Here's how the part is built. I have some questions about the finished solid (model axes, mm). A direction names the side the tool comes from. Coordinates: 2 decimals unless noted, no trailing zeros. Write each loop counter-clockwise with the first axis right and the second up, starting at its lowest first coordinate (ties: lowest second). Pieces come first, ordered by that corner, then holes. Notation, with made-up numbers: M 13.5,27.25 L 69.5,27.25 A31 ccw 69.5,58.25 Z; hole C 14.25,1.5 d4. An arc over 180 degrees is marked long. Use one line per item in the form item = value. Start each with the question number.
1. I want a section at A-A, the plane y = 3. List the corners of the cut face in (x, z) for me, plus the area to 3 significant figures.
2. Thinking about a two-plate mould opening in Y: for faces 1 (the face through (35.6, 25.926, 0)), 2 (the face through (40, 8, 0)), 3 (the face through (32, 0, 0)), which applies, released by +Y, released by -Y, zero draft, split by the parting line, or undercut?
3. I want a section at D-D, the plane x = 27. List the corners of the cut face in (y, z) for me.
4. On a 3-axis mill with a long thin cutter (end or side, diameter ignored), from which of +Z, -Z, +X, -X, +Y, -Y can I reach the whole of each face in a straight line? I mean faces 4 (the face through (38, 15.926, 0)), 5 (the face through (4.926, 25, 0)), 6 (the face through (20, 20, -1.5)). Say none if no direction works.
5. I'm going to push a flat-ended pin straight in: pin 1 Ø1.5 at (y, z) = (22.5, 0) entering from +X. Where does the tip first touch, or does it pass through?
6. Please list where these lines run through material, in increasing order: line 1 along Y through (x, z) = (4.5, 0.7); line 2 along Y through (x, z) = (15, -1.25); line 3 along X through (y, z) = (33, -1.25). Write a range as [from, to].
7. I want a section at B-B, the plane x = 32. List the corners of the cut face in (y, z) for me, plus the area to 3 significant figures.
8. I want a section at C-C, the plane y = 27. List the corners of the cut face in (x, z) for me, plus the area to 3 significant figures.
Autodesk Inventor part; units mm, degrees
ref_plane "YZ Plane" through (0, 0, 0) normal (1, 0, 0) x (0, 1, 0)
ref_plane "XZ Plane" through (0, 0, 0) normal (0, 1, 0) x (-1, 0, 0)
ref_plane "XY Plane" through (0, 0, 0) normal (0, 0, 1) x (1, 0, 0)
sketch "스케치1" plane through (0, 0, 0) normal (0, 0, 1) x (1, 0, 0)
  line L0 (40, 40) -> (25, 40)
  line L1 (15, 40) -> (0, 40)
  line L2 (16, 40) -> (16, 35)
  line L3 (16, 35) -> (14, 35)
  line L4 (14, 35) -> (14, 36)
  line L5 (14, 36) -> (11, 36)
  line L6 (11, 36) -> (11, 31)
  line L7 (11, 31) -> (14, 28)
  line L8 (11, 31) -> (20.81, 31) construction
  line L9 (14, 28) -> (20, 28)
  line L10 (24, 40) -> (24, 35)
  line L11 (24, 35) -> (26, 35)
  line L12 (26, 35) -> (26, 36)
  line L13 (26, 36) -> (29, 36)
  line L14 (29, 36) -> (29, 31)
  line L15 (29, 31) -> (26, 28)
  line L16 (29, 31) -> (19.19, 31) construction
  line L17 (26, 28) -> (20, 28)
  line L18 (-0.0744, 15.9256) -> (4.9256, 15.9256)
  line L19 (-0.0744, 23.9256) -> (4.9256, 23.9256)
  line L20 (4.9256, 23.9256) -> (4.9256, 25.9256)
  line L21 (11.9256, 25.9256) -> (11.9256, 19.9256)
  line L22 (8.9256, 28.9256) -> (8.9256, 19.1155) construction
  line L23 (8.9256, 28.9256) -> (11.9256, 25.9256)
  line L24 (3.9256, 28.9256) -> (8.9256, 28.9256)
  line L25 (3.9256, 25.9256) -> (3.9256, 28.9256)
  line L26 (4.9256, 25.9256) -> (3.9256, 25.9256)
  line L27 (4.9256, 15.9256) -> (4.9256, 13.9256)
  line L28 (11.9256, 13.9256) -> (11.9256, 19.9256)
  line L29 (4.9256, 13.9256) -> (3.9256, 13.9256)
  line L30 (8.9256, 10.9256) -> (11.9256, 13.9256)
  line L31 (8.9256, 10.9256) -> (8.9256, 20.7356) construction
  line L32 (3.9256, 13.9256) -> (3.9256, 10.9256)
  line L33 (3.9256, 10.9256) -> (8.9256, 10.9256)
  line L34 (24, -0.1488) -> (24, 4.8512)
  line L35 (16, -0.1488) -> (16, 4.8512)
  line L36 (16, 4.8512) -> (14, 4.8512)
  line L37 (14, 11.8512) -> (20, 11.8512)
  line L38 (11, 8.8512) -> (20.81, 8.8512) construction
  line L39 (11, 8.8512) -> (14, 11.8512)
  line L40 (11, 3.8512) -> (11, 8.8512)
  line L41 (14, 3.8512) -> (11, 3.8512)
  line L42 (14, 4.8512) -> (14, 3.8512)
  line L43 (24, 4.8512) -> (26, 4.8512)
  line L44 (26, 11.8512) -> (20, 11.8512)
  line L45 (26, 4.8512) -> (26, 3.8512)
  line L46 (29, 8.8512) -> (26, 11.8512)
  line L47 (29, 8.8512) -> (19.19, 8.8512) construction
  line L48 (26, 3.8512) -> (29, 3.8512)
  line L49 (29, 3.8512) -> (29, 8.8512)
  line L50 (40.0744, 23.9256) -> (35.0744, 23.9256)
  line L51 (40.0744, 15.9256) -> (35.0744, 15.9256)
  line L52 (35.0744, 15.9256) -> (35.0744, 13.9256)
  line L53 (28.0744, 13.9256) -> (28.0744, 19.9256)
  line L54 (31.0744, 10.9256) -> (31.0744, 20.7356) construction
  line L55 (31.0744, 10.9256) -> (28.0744, 13.9256)
  line L56 (36.0744, 10.9256) -> (31.0744, 10.9256)
  line L57 (36.0744, 13.9256) -> (36.0744, 10.9256)
  line L58 (35.0744, 13.9256) -> (36.0744, 13.9256)
  line L59 (35.0744, 23.9256) -> (35.0744, 25.9256)
  line L60 (28.0744, 25.9256) -> (28.0744, 19.9256)
  line L61 (35.0744, 25.9256) -> (36.0744, 25.9256)
  line L62 (31.0744, 28.9256) -> (28.0744, 25.9256)
  line L63 (31.0744, 28.9256) -> (31.0744, 19.1155) construction
  line L64 (36.0744, 25.9256) -> (36.0744, 28.9256)
  line L65 (36.0744, 28.9256) -> (31.0744, 28.9256)
  line L66 (11, 20) -> (11.9256, 20)
  line L67 (28.0744, 20) -> (29, 20)
  line L68 (20, 3.8512) -> (20, 4.8512)
  line L69 (20, 35) -> (20, 36)
  line L70 (15, 40) -> (16, 40)
  line L71 (24, 40) -> (25, 40)
  line L72 (0, 40) -> (0, 23.9256)
  line L73 (0, 15.9256) -> (0, 0)
  line L74 (40, 0) -> (40, 15.9256)
  line L75 (40, 23.9256) -> (40, 40)
  line L76 (0, 0) -> (16, 0)
  line L77 (24, 0) -> (40, 0)
  point P0 (25, 38)
  point P1 (20, 19.9256)
  point P2 (15, 35)
  point P3 (25, 35)
  point P4 (4.9256, 24.9256)
  point P5 (4.9256, 14.9256)
  point P6 (15, 4.8512)
  point P7 (25, 4.8512)
  point P8 (35.0744, 14.9256)
  point P9 (35.0744, 24.9256)
  dimension "d0" = 40
  dimension "d1" = 40
  dimension "d14" = 2
  dimension "d15" = 5
  dimension "d16" = 1
  dimension "d17" = 3
  dimension "d18" = 5
  dimension "d19" = 45
  dimension "d21" = 7
  dimension "d24" = 360
extrude "돌출1" add sketch "스케치1" along normal mid plane 3
properties part number "79" material "철, 회색"
Answer list:
q1.outline = M 0,-1.5 L 16,-1.5 L 16,1.5 L 0,1.5 Z; M 24,-1.5 L 40,-1.5 L 40,1.5 L 24,1.5 Z
q1.area = 96.0 mm²
q2.face_1 = undercut
q2.face_2 = zero draft
q2.face_3 = released by -Y
q3.outline = M 0,-1.5 L 3.85,-1.5 L 3.85,1.5 L 0,1.5 Z; M 10.85,-1.5 L 29,-1.5 L 29,1.5 L 10.85,1.5 Z; M 36,-1.5 L 40,-1.5 L 40,1.5 L 36,1.5 Z
q4.face_4 = +Z, -Z, +X
q4.face_5 = +Z, -Z
q4.face_6 = -Z, +X, -X, +Y, -Y
q5.pin_1 = 28.07
q6.line_1 = [0, 10.93], [13.93, 15.93], [23.93, 25.93], [28.93, 40]
q6.line_2 = [0, 4.85], [11.85, 28], [35, 40]
q6.line_3 = [0, 11], [29, 40]
q7.outline = M 0,-1.5 L 10.93,-1.5 L 10.93,1.5 L 0,1.5 Z; M 28.93,-1.5 L 40,-1.5 L 40,1.5 L 28.93,1.5 Z
q7.area = 66.0 mm²
q8.outline = M 0,-1.5 L 3.93,-1.5 L 3.93,1.5 L 0,1.5 Z; M 10.85,-1.5 L 29.15,-1.5 L 29.15,1.5 L 10.85,1.5 Z; M 36.07,-1.5 L 40,-1.5 L 40,1.5 L 36.07,1.5 Z
q8.area = 78.4 mm²
